```python
from build123d import *

# Parameters (mm, degrees)
F0_W     = 600
F0_H     = 360
F1_DEPTH = 570
F3_DEPTH = 120
F5_DEPTH = 360.001


with BuildPart() as f1:
    # F0 (on Top) → F1 (new body)
    with BuildSketch(Plane.XY):
        Rectangle(F0_W, F0_H)
    extrude(amount=F1_DEPTH)

    # F2 (on face) → F3 (join)
    with BuildSketch(Plane.XY.offset(570)):
        Polygon((-300, 39.58638), (-187.376666, 180), (-300, 180), align=None)
        Polygon((300, 180), (160.513226, 180), (300, 66.23076), align=None)
    extrude(amount=F3_DEPTH)

    # F4 (on face) → F5 (cut, through all)
    with BuildSketch(Plane.XZ.offset(180)):
        Polygon((0, 0), (100, 0), (100, 250), (-100, 250), (-100, 0), align=None)
    extrude(amount=-F5_DEPTH, mode=Mode.SUBTRACT)


solid = f1.part
```
Source: CAD feature listing. Evaluate the final solid. Frame: model axes, mm. A direction names the side the tool comes from. Give positions to 0.01 mm unless a question says otherwise; leave off trailing zeros. Write each loop counter-clockwise with the first axis right and the second up, starting at its lowest first coordinate (ties: lowest second). Pieces come first, ordered by that corner, then holes. Notation, with made-up numbers: (29, 36) - (65, 36) arc R22 cw to (65, 56) - close; hole circle Ø3 at (43.25, 17.25). An arc over 180 degrees is marked (long way). One line per item, written item: value. Start each with the question number.
Q1. Section query A-A, the plane z = 43.5. Return the cut outline in (x, y), then the cut area to 3 significant figures.
Q2. Section query B-B, the plane y = -44. Return the cut outline in (x, z).
Q3. Section query D-D, the plane y = 122. Return the cut outline in (x, z).
Q4. First-contact query: pin 1 Ø10 at (x, y) = (-70.5, 83) entering from +Z. Flat tip, straight axial feed; report the tip coordinate or a pass-through.
Q5. Draft query along X for faces 4 (the face through (260, 149, 690)), 5 (the face through (300, -3, 264)), 6 (the face through (-244.477, 108.81, 629.16)). Return one class per face: +X half, -X half, draft (parallel to the pull), parting line (faces both ways), or undercut.
Q6. Material intervals for probe 1 along X at (y, z) = (-12.5, 185); probe 2 along Z at (x, y) = (59.5, -130.5); probe 3 along Z at (x, y) = (-150, -8), sorted ascending. Write a range as from..to.
Q7. Section query C-C, the plane x = -54.5. Return the cut outline in (y, z).
Q8. Set-up query: faces 1 (the face through (-4, 3, 570)), 2 (the face through (-100, -3, 127)), 3 (the face through (-300, 3, 340)). Return all of +Z, -Z, +X, -X, +Y, -Y with unobstructed straight access to the full face (end or side cutting, diameter ignored); none if empty.
Answer:
1. outline: (-300, -180) - (-100, -180) - (-100, 180) - (-300, 180) - close; (100, -180) - (300, -180) - (300, 180) - (100, 180) - close
1. area: 144,000 mm2
2. outline: (-300, 0) - (-100, 0) - (-100, 250) - (100, 250) - (100, 0) - (300, 0) - (300, 570) - (-300, 570) - close
3. outline: (-300, 0) - (-100, 0) - (-100, 250) - (100, 250) - (100, 0) - (300, 0) - (300, 690) - (231.62, 690) - (231.62, 570) - (-233.9, 570) - (-233.9, 690) - (-300, 690) - close
4. pin 1: stops at z = 570
5. face 4: draft
5. face 5: +X half
5. face 6: undercut
6. probe 1: x = -300..-100, 100..300
6. probe 2: z = 250..570
6. probe 3: z = 0..570
7. outline: (-180, 250) - (180, 250) - (180, 570) - (-180, 570) - close
8. face 1: +Z, -Y
8. face 2: -Z, +Y, -Y
8. face 3: +Z, -Z, -X, +Y, -Y
